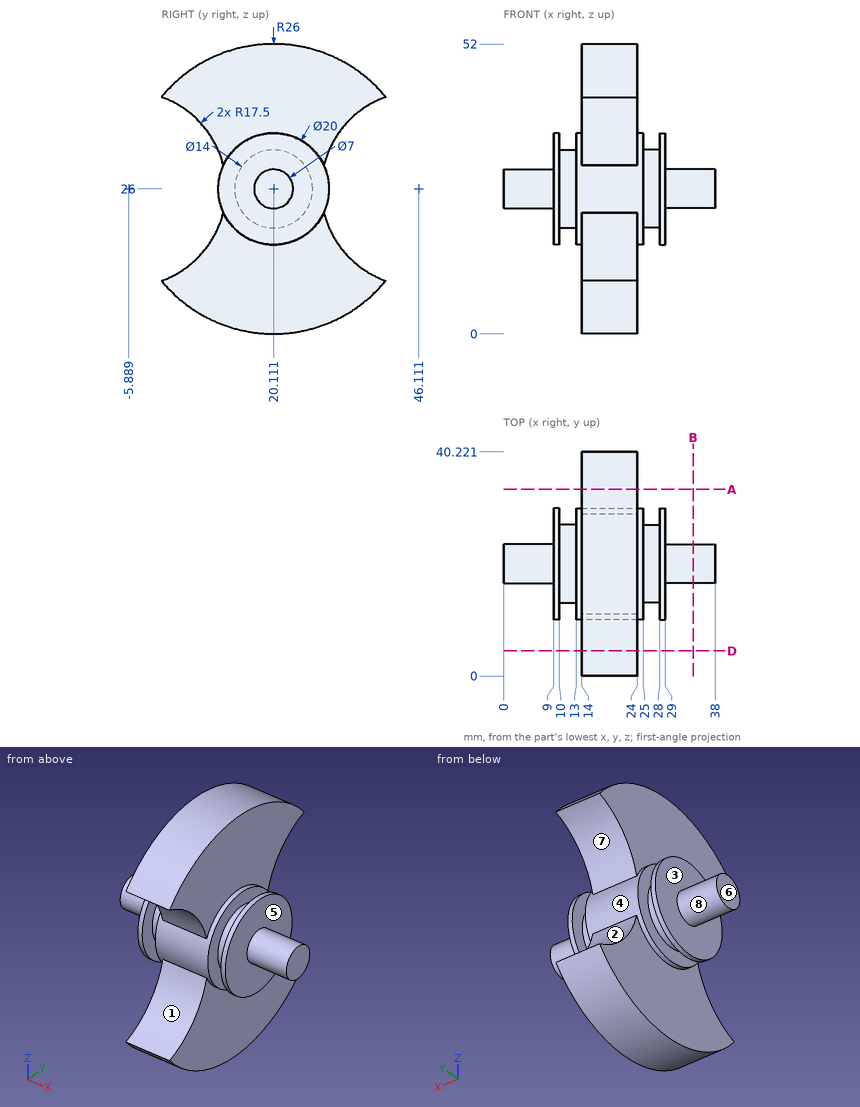
Geometry: see drawing. Coordinates: mm, zero at the bounding-box minimum. A direction names the side the tool comes from. Give positions to 0.01 mm unless a question says otherwise; leave off trailing zeros. Write each loop counter-clockwise with the first axis right and the second up, starting at its lowest first coordinate (ties: lowest second). Pieces come first, ordered by that corner, then holes. Notation, with made-up numbers: (-14, 62) - (-1, 62) arc R13 ccw to (-1, 73) - close; hole circle Ø7 at (-9.5, -11). An arc over 180 degrees is marked (long way). Return JSON: item names as keys, results as strings. Group by question number.
1) Set-up query: the marked faces 1, 2, 3, 4 and 5. Return all of +Z, -Z, +X, -X, +Y, -Y with unobstructed straight access to the full face (end or side cutting, diameter ignored); none if empty.
2) First-contact query: P1, Ø11, axis at y = 13.5, z = 12.5, coming from the -X side; P2, Ø3, axis at y = 21.5, z = 40, coming from the -X side; P3, Ø16, axis at y = 16.5, z = 25.5, coming from the +X side; P4, Ø11, axis at y = 19.5, z = 9, coming from the +X side. Flat tips, straight axial feed; report the tip coordinate or a pass-through.
3) Section D-D on y = 4.5. Return the cut outline in (x, z).
4) Line query: line 1 (X direction, y = 11, z = 14); line 2 (Y direction, x = 17, z = 2) (1 decimal); line 3 (X direction, y = 24, z = 28). Output: solid intervals per line, ascending.
5) Section A-A on y = 33.5. Return the cut outline in (x, z), plus the area to 3 significant figures.
6) Mould query, pull axis Z, two halves, no side actions, for the marked faces 6, 7 and 8. Classes: released by +Z, released by -Z, zero draft, split by the parting line, or undercut.
7) Section B-B on x = 34. Return the cut outline in (y, z), plus the area to 3 significant figures.
Filled in:
{
 "1": {"face 1": "+X, -X, -Y", "face 2": "+X, -X, +Y", "face 3": "-X", "face 4": "none", "face 5": "+X"},
 "2": {"P1": "stops at x = 9", "P2": "stops at x = 14", "P3": "stops at x = 38", "P4": "stops at x = 24"},
 "3": {"outline": "(14, 5.21) - (24, 5.21) - (24, 11.92) - (14, 11.92) - close; (14, 40.08) - (24, 40.08) - (24, 46.79) - (14, 46.79) - close"},
 "4": {"line 1": "x = 14 to 24", "line 2": "y = 10.1 to 30.1", "line 3": "x = 9 to 29"},
 "5": {"outline": "(14, 3.71) - (24, 3.71) - (24, 13.87) - (14, 13.87) - close; (14, 38.13) - (24, 38.13) - (24, 48.29) - (14, 48.29) - close", "area": "203 mm^2"},
 "6": {"face 6": "zero draft", "face 7": "undercut", "face 8": "split by the parting line"},
 "7": {"outline": "circle Ø7 at (20.11, 26)", "area": "38.5 mm^2"}
}
